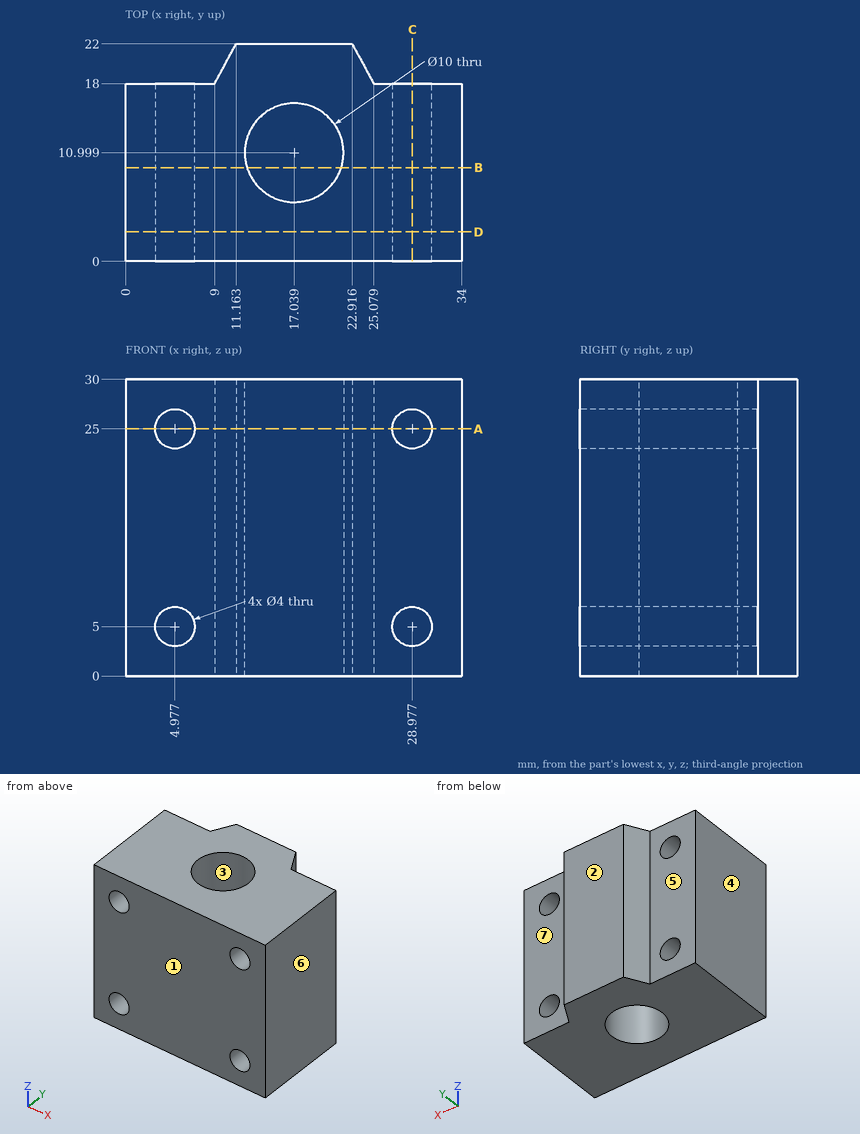
Print and shaded views of the part. All mm, measured from the part's lowest x, y and z. A direction names the side the tool comes from. Give positions to 0.01 mm unless a question says otherwise; leave off trailing zeros. Write each loop counter-clockwise with the first axis right and the second up, starting at its lowest first coordinate (ties: lowest second). Pieces come first, ordered by that corner, then holes. Notation, with made-up numbers: M 20,-28 L 34,-28 A14 ccw 34,-6 Z; hole C 66,42.5 d8. An arc over 180 degrees is marked long. Use a Markdown table: item, result.
1) Cut at C-C (x = 29). List the corners of the cut face in (y, z).
Responses:
| item | result |
|---|---|
| outline | M 0,0 L 18,0 L 18,3 L 0,3 Z; M 0,7 L 18,7 L 18,23 L 0,23 Z; M 0,27 L 18,27 L 18,30 L 0,30 Z |
2) Cut at B-B (y = 9.5). List the corners of the cut face in (x, z).
Responses:
| item | result |
|---|---|
| outline | M 0,0 L 12.27,0 L 12.27,30 L 0,30 Z; M 21.81,0 L 34,0 L 34,30 L 21.81,30 Z; hole C 4.98,5 d4; hole C 4.98,25 d4; hole C 28.98,5 d4; hole C 28.98,25 d4 |
3) Cut at D-D (y = 3). List the corners of the cut face in (x, z).
Responses:
| item | result |
|---|---|
| outline | M 0,0 L 34,0 L 34,30 L 0,30 Z; hole C 4.98,5 d4; hole C 4.98,25 d4; hole C 28.98,5 d4; hole C 28.98,25 d4 |
4) Tool access for the marked faces 5, 6 and 7: list every direction of +Z, -Z, +X, -X, +Y, -Y with a clear straight run to the whole face (end or side of a thin tool).
Responses:
| item | result |
|---|---|
| face 5 | +Z, -Z, -X, +Y |
| face 6 | +Z, -Z, +X, +Y, -Y |
| face 7 | +Z, -Z, +X, +Y |
5) Cut at A-A (z = 25). List the corners of the cut face in (x, y).
Responses:
| item | result |
|---|---|
| outline | M 0,0 L 2.98,0 L 2.98,18 L 0,18 Z; M 6.98,0 L 26.98,0 L 26.98,18 L 25.08,18 L 22.92,22 L 11.16,22 L 9,18 L 6.98,18 Z; M 30.98,0 L 34,0 L 34,18 L 30.98,18 Z; hole C 17.04,11 d10 |
6) Drill centre lines: line 1 (X direction, y = 5.5, z = 25); line 2 (X direction, y = 15.5, z = 5.5) (1 decimal); line 3 (Z direction, x = 4, y = 5.5) (1 decimal). Where is each one in solid material? Low to high. Write a range as from..to.
Responses:
| item | result |
|---|---|
| line 1 | x = 0..2.98, 6.98..26.98, 30.98..34 |
| line 2 | x = 0..3, 6.9..14.9, 19.2..27, 30.9..34 |
| line 3 | z = 0..3.3, 6.7..23.3, 26.7..30 |
7) Pull direction Y, two halves, no side cores. Call the marked faces 1, 2, 3 and 4: +Y half, -Y half, draft (parallel to the pull), parting line (faces both ways), or undercut.
Responses:
| item | result |
|---|---|
| face 1 | -Y half |
| face 2 | +Y half |
| face 3 | undercut |
| face 4 | draft |
8) Pin check, flat tips, straight feed: pin 1 (7 mm diameter, centred on x = 31, z = 22, fed in from +Y); pin 2 (8 mm diameter, centred on x = 17.04, y = 11, fed in from -Z). Stop position of each tip, or through.
Responses:
| item | result |
|---|---|
| pin 1 | stops at y = 18 |
| pin 2 | passes through |
